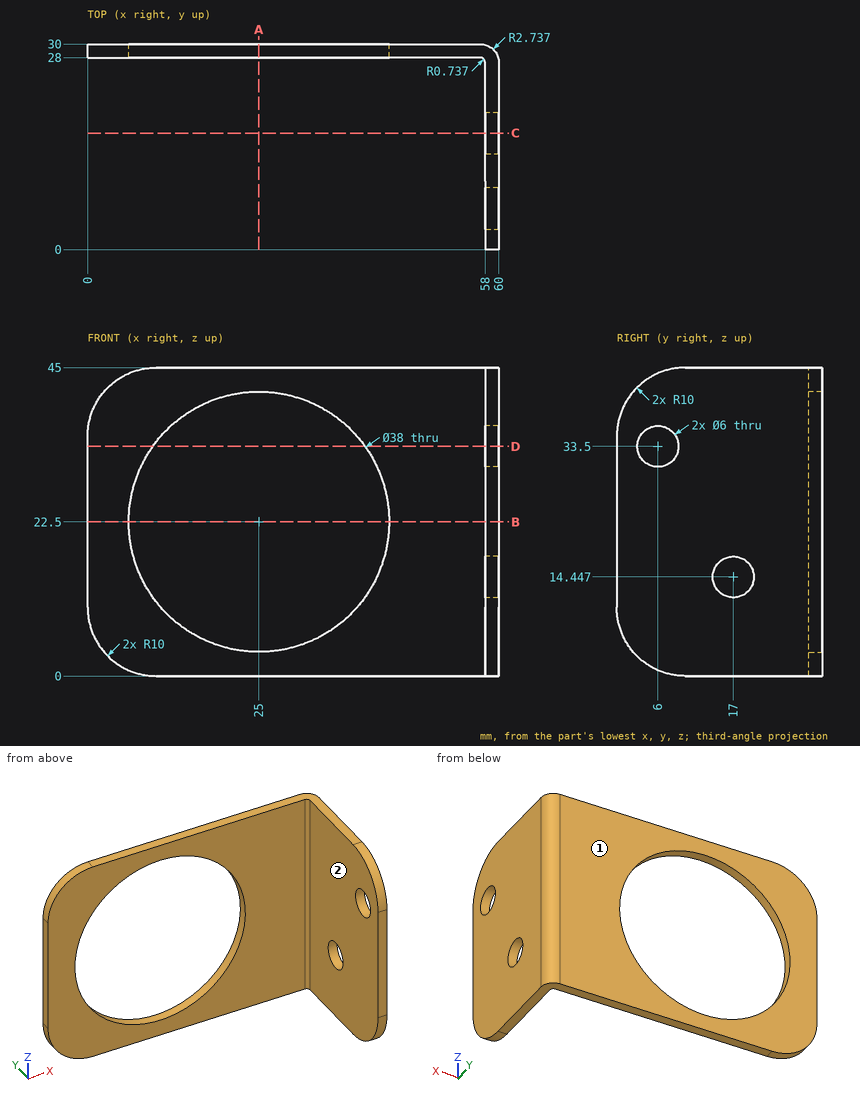
Input: dimensioned drawing with shaded views. Units: mm. Origin: part minimum x, y, z. A direction names the side the tool comes from. Give positions to 0.01 mm unless a question says otherwise; leave off trailing zeros. Order: outer loops, then holes, each group sorted by start corner. A loop starts at its lowest first (then second) coordinate and runs counter-clockwise, first axis right, second up. Notation, with made-up numbers: (45, 6) -> (91, 6) arc R22 ccw to (91, 27) -> close; hole circle Ø1 at (36, -12.75). An arc over 180 degrees is marked (long way). Use a Markdown table: item, result.
1) Section query C-C, the plane y = 17. Return the cut outline in (x, z).
Answer list:
| item | result |
|---|---|
| outline | (58, 0) -> (60, 0) -> (60, 11.45) -> (58, 11.45) -> close; (58, 17.45) -> (60, 17.45) -> (60, 45) -> (58, 45) -> close |
2) Ray query, line 1 along Z through (x, y) = (59.25, 17); line 2 along Y through (x, z) = (49, 5.5); line 3 along X through (y, z) = (26.25, 41). Return the intervals inside material, ascending. Write a range as [from, to].
Answer list:
| item | result |
|---|---|
| line 1 | [0, 11.45], [17.45, 45] |
| line 2 | [28, 30] |
| line 3 | [58, 60] |
3) Section query B-B, the plane z = 22.5. Return the cut outline in (x, y).
Answer list:
| item | result |
|---|---|
| outline | (0, 28) -> (6, 28) -> (6, 30) -> (0, 30) -> close; (44, 28) -> (57.26, 28) arc R0.74 cw to (58, 27.26) -> (58, 0) -> (60, 0) -> (60, 27.26) arc R2.74 ccw to (57.26, 30) -> (44, 30) -> close |
4) Section query D-D, the plane z = 33.5. Return the cut outline in (x, y).
Answer list:
| item | result |
|---|---|
| outline | (0, 28) -> (9.51, 28) -> (9.51, 30) -> (0, 30) -> close; (40.49, 28) -> (57.26, 28) arc R0.74 cw to (58, 27.26) -> (58, 9) -> (60, 9) -> (60, 27.26) arc R2.74 ccw to (57.26, 30) -> (40.49, 30) -> close; (58, 0) -> (60, 0) -> (60, 3) -> (58, 3) -> close |
5) Reachability of the marked faces 1 and 2 from +Z, -Z, +X, -X, +Y, -Y: full face, straight path, thin tool, end or side. Return the list, or none.
Answer list:
| item | result |
|---|---|
| face 1 | +Z, -Z, +X, -X, +Y |
| face 2 | +Z, -Z, -X, -Y |
6) Contact query for flat-ended pins moving along their axis: P1, Ø2, axis at x = 44, z = 4.5, coming from the -Y side; P2, Ø5, axis at y = 6, z = 33.5, coming from the +X side; P3, Ø3, axis at y = 8.5, z = 28.5, coming from the -X side. Output: stop coordinate, or through.
Answer list:
| item | result |
|---|---|
| P1 | y = 28 |
| P2 | through |
| P3 | x = 58 |
7) Section query A-A, the plane x = 25. Return the cut outline in (y, z).
Answer list:
| item | result |
|---|---|
| outline | (28, 0) -> (30, 0) -> (30, 3.5) -> (28, 3.5) -> close; (28, 41.5) -> (30, 41.5) -> (30, 45) -> (28, 45) -> close |
